```python
from build123d import *

# Parameters (mm, degrees)
F0_R     = 12.7
F1_DEPTH = 25.4
F3_DEPTH = 25.401
F4_DEPTH = 11.0998
F6_DEPTH = 9.525


with BuildPart() as f1:
    # F0 (on Front) → F1 (new body)
    with BuildSketch(Plane.XZ):
        Circle(F0_R)
    extrude(amount=F1_DEPTH)

    # F2 (on face) → F3 (cut, through all)
    with BuildSketch(Plane.XZ.offset(25.4)):
        with BuildLine():
            ThreePointArc((4.7625, 0), (3.367596, 3.367596), (0, 4.7625))
            ThreePointArc((0, 4.7625), (-3.367596, 3.367596), (-4.7625, 0))
            ThreePointArc((-4.7625, 0), (-3.367596, -3.367596), (0, -4.7625))
            ThreePointArc((0, -4.7625), (3.367596, -3.367596), (4.7625, 0))
        make_face()
    extrude(amount=-F3_DEPTH, mode=Mode.SUBTRACT)

    # F2 (on face) → F4 (cut)
    with BuildSketch(Plane.XZ.offset(25.4)):
        with BuildLine():
            Line((0, 4.7625), (-4.7625, 4.7625))
            Line((-4.7625, 4.7625), (-4.7625, 0))
            ThreePointArc((-4.7625, 0), (-3.367596, 3.367596), (0, 4.7625))
        make_face()
        with BuildLine():
            Line((4.7625, 4.7625), (0, 4.7625))
            ThreePointArc((0, 4.7625), (3.367596, 3.367596), (4.7625, 0))
            Line((4.7625, 0), (4.7625, 4.7625))
        make_face()
        with BuildLine():
            ThreePointArc((0, -4.7625), (-3.367596, -3.367596), (-4.7625, 0))
            Line((-4.7625, 0), (-4.7625, -4.7625))
            Line((-4.7625, -4.7625), (0, -4.7625))
        make_face()
        with BuildLine():
            Line((4.7625, -4.7625), (4.7625, 0))
            ThreePointArc((4.7625, 0), (3.367596, -3.367596), (0, -4.7625))
            Line((0, -4.7625), (4.7625, -4.7625))
        make_face()
    extrude(amount=-F4_DEPTH, mode=Mode.SUBTRACT)

    # F5 (on face) → F6 (cut)
    with BuildSketch(Plane.XZ.offset(25.4)):
        Polygon((-12.624906, 1.143208), (-7.3025, -10.361885), (5.322406, -11.505093), (12.624906, -1.143208), (7.3025, 10.361885), (-5.322406, 11.505093), align=None)
    extrude(amount=-F6_DEPTH, mode=Mode.SUBTRACT)


solid = f1.part
```
Part model, mm, in its own coordinate system. A direction names the side the tool comes from. Coordinates: 2 decimals unless noted, no trailing zeros. Order: outer loops, then holes, each group sorted by start corner. A loop starts at its lowest first (then second) coordinate and runs counter-clockwise, first axis right, second up. Notation, with made-up numbers: (1.25, 24.5) - (11.25, 24.5) arc R16 ccw to (11.25, 52.5) - close; hole circle Ø1 at (67, -24). An arc over 180 degrees is marked (long way). Return JSON: item names as keys, results as strings. Group by question number.
Item 1: Which spindle directions (+Z, -Z, +X, -X, +Y, -Y) get a long thin tool onto all of the face, cutting with end or side? Do faces 4 (the face through (5, 0, 0)), 5 (the face through (0, -15.875, 5)). Say none if no direction does.
Item 2: Drill centre lines: probe 1 along Z at (x, y) = (0.25, -10.75); probe 2 along Y at (x, z) = (-3.5, -6) (3 decimals); probe 3 along X at (y, z) = (-21.5, -6.5). Where is each one in solid material? Low to high. Write a range as from..to.
Item 3: Cut at D-D (z = 7.5). List the corners of the cut face in (x, y) (3 decimals), plus the area to 3 significant figures.
Item 4: Pull direction Z, two halves, no side cores. Call faces 1 (the face through (-2.75, -12.52, -12.4)), 2 (the face through (-1, -25.4, -11.2)), 3 (the face through (-4, -14.3, 4)): pulls with the +Z half, pulls with the -Z half, needs draft (parallel to the pull), parting line crosses it, or undercut.
Item 5: Pin check, flat tips, straight feed: pin 1 (1.5 mm diameter, centred on x = -1, y = -9.5, fed in from -Z); pin 2 (1.7 mm diameter, centred on x = -2.5, y = -15, fed in from -Z); pin 3 (5 mm diameter, centred on x = -3.5, z = -2.5, fed in from -Y) (3 decimals). Stop position of each tip, or through.
Item 6: Cut at A-A (y = -5). List the corners of the cut face in (x, z) (1 decimal).
Check values:
{
 "1": {"face 4": "+Z, -Z, +X, -X, +Y", "face 5": "-Y"},
 "2": {"probe 1": "z = -12.7..-4.76, 4.76..12.7", "probe 2": "y = -15.875..0", "probe 3": "x = -10.91..-9.09, 8.85..10.91"},
 "3": {"outline": "(-10.249, -25.4) - (-8.145, -25.4) - (-8.145, -15.875) - (8.626, -15.875) - (8.626, -25.4) - (10.249, -25.4) - (10.249, 0) - (-10.249, 0) - close", "area": "361 mm2"},
 "4": {"face 1": "parting line crosses it", "face 2": "needs draft", "face 3": "undercut"},
 "5": {"pin 1": "stops at z = -12.7", "pin 2": "stops at z = -12.59", "pin 3": "stops at y = -15.875"},
 "6": {"outline": "circle Ø25.4 at (0, 0); hole circle Ø9.5 at (0, 0)"}
}
